from build123d import *

# Parameters (mm, degrees)
F0_W     = 156.21
F0_H     = 80.01
F1_DEPTH = 8.46582
F2_W     = 25.4
F2_H     = 80.01
F3_DEPTH = 1.27
F4_DEPTH = 2.54
F2_W_2   = 27.305
F5_DEPTH = 1.27
F6_DEPTH = 2.54
F7_DEPTH = 1.27
F8_DEPTH = 2.54


with BuildPart() as f1:
    # F0 (on Top) → F1 (new body)
    with BuildSketch(Plane.XY):
        Rectangle(F0_W, F0_H)
    extrude(amount=F1_DEPTH)

    # F2 (on face) → F3 (cut)
    with BuildSketch(Plane.XY.offset(8.46582)):
        with Locations((-65.405, 0)):
            Rectangle(F2_W, F2_H)
    extrude(amount=-F3_DEPTH, mode=Mode.SUBTRACT)

    # F2 (on face) → F4 (cut)
    with BuildSketch(Plane.XY.offset(8.46582)):
        with Locations((-40.005, 0)):
            Rectangle(F2_W, F2_H)
    extrude(amount=-F4_DEPTH, mode=Mode.SUBTRACT)

    # F2 (on face) → F5 (cut)
    with BuildSketch(Plane.XY.offset(8.46582)):
        with Locations((-13.6525, 0)):
            Rectangle(F2_W_2, F2_H)
    extrude(amount=-F5_DEPTH, mode=Mode.SUBTRACT)

    # F2 (on face) → F6 (cut)
    with BuildSketch(Plane.XY.offset(8.46582)):
        with Locations((12.7, 0)):
            Rectangle(F2_W, F2_H)
    extrude(amount=-F6_DEPTH, mode=Mode.SUBTRACT)

    # F2 (on face) → F7 (cut)
    with BuildSketch(Plane.XY.offset(8.46582)):
        with Locations((38.1, 0)):
            Rectangle(F2_W, F2_H)
    extrude(amount=-F7_DEPTH, mode=Mode.SUBTRACT)

    # F2 (on face) → F8 (cut)
    with BuildSketch(Plane.XY.offset(8.46582)):
        with Locations((64.4525, 0)):
            Rectangle(F2_W_2, F2_H)
    extrude(amount=-F8_DEPTH, mode=Mode.SUBTRACT)


solid = f1.part
Can you work these out from the model? Positions are in its coordinate system, mm. A direction names the side the tool comes from. Coordinates: 2 decimals unless noted, no trailing zeros. Loops run counter-clockwise (first coordinate to the right, second up) from the corner with the lowest first, then second, coordinate; pieces in that order, holes last. Notation, with made-up numbers: (79, 40.25) - (131, 40.25) arc R11 ccw to (131, 58.25) - close; hole circle Ø6 at (1, -35.75). An arc over 180 degrees is marked (long way). Put each result on its own line as item: value. Start each with the question number.
Item 1: If I drill on line 1 along X through (y, z) = (8, 6.5) (3 decimals); line 2 along Z through (x, y) = (16, 8.5), over which ranges is the centre line in solid material (lowest first)?
Item 2: Suppose I cut it at B-B (x = 18.5). Please give me the cut outline in (y, z) (3 decimals).
Item 3: Suppose I cut it at A-A (y = -5). Please give me the cut outline in (x, z) (3 decimals), and give its area (3 significant figures).
Item 4: For pin 1 (7.5 mm diameter, centred on x = -42.5, y = 18.5, fed in from +Z); pin 2 (1.4 mm diameter, centred on y = -17, z = 7, fed in from +X), each with a flat end and sliding along its axis, tell me the tip position at first contact or that it passes through.
Item 5: Which directions (+Z, -Z, +X, -X, +Y, -Y) give clear straight access to the entire face, cutting with the end or side of a thin tool? Please do faces 1 (the face through (13, 1, 5.926)), 2 (the face through (-66, 1, 7.196)), 3 (the face through (64, 1, 5.926)).
Item 6: If we mould it in two halves opening along X, with no side actions, what happens to faces 4 (the face through (-1, 1, 0)), 5 (the face through (-40, 1, 5.926)), 6 (the face through (78.105, -1, 3))? For each: +X half, -X half, draft (parallel to the pull), parting line (faces both ways), or undercut.
Here are the results:
1. line 1: -78.105 to -52.705, -27.305 to 0, 25.4 to 50.8
1. line 2: 0 to 5.93
2. outline: (-40.005, 0) - (40.005, 0) - (40.005, 5.926) - (-40.005, 5.926) - close
3. outline: (-78.105, 0) - (78.105, 0) - (78.105, 5.926) - (50.8, 5.926) - (50.8, 7.196) - (25.4, 7.196) - (25.4, 5.926) - (0, 5.926) - (0, 7.196) - (-27.305, 7.196) - (-27.305, 5.926) - (-52.705, 5.926) - (-52.705, 7.196) - (-78.105, 7.196) - close
3. area: 1,020 mm²
4. pin 1: z = 5.93
4. pin 2: x = 50.8
5. face 1: +Z, +Y, -Y
5. face 2: +Z, +X, -X, +Y, -Y
5. face 3: +Z, +X, +Y, -Y
6. face 4: draft
6. face 5: undercut
6. face 6: +X half
